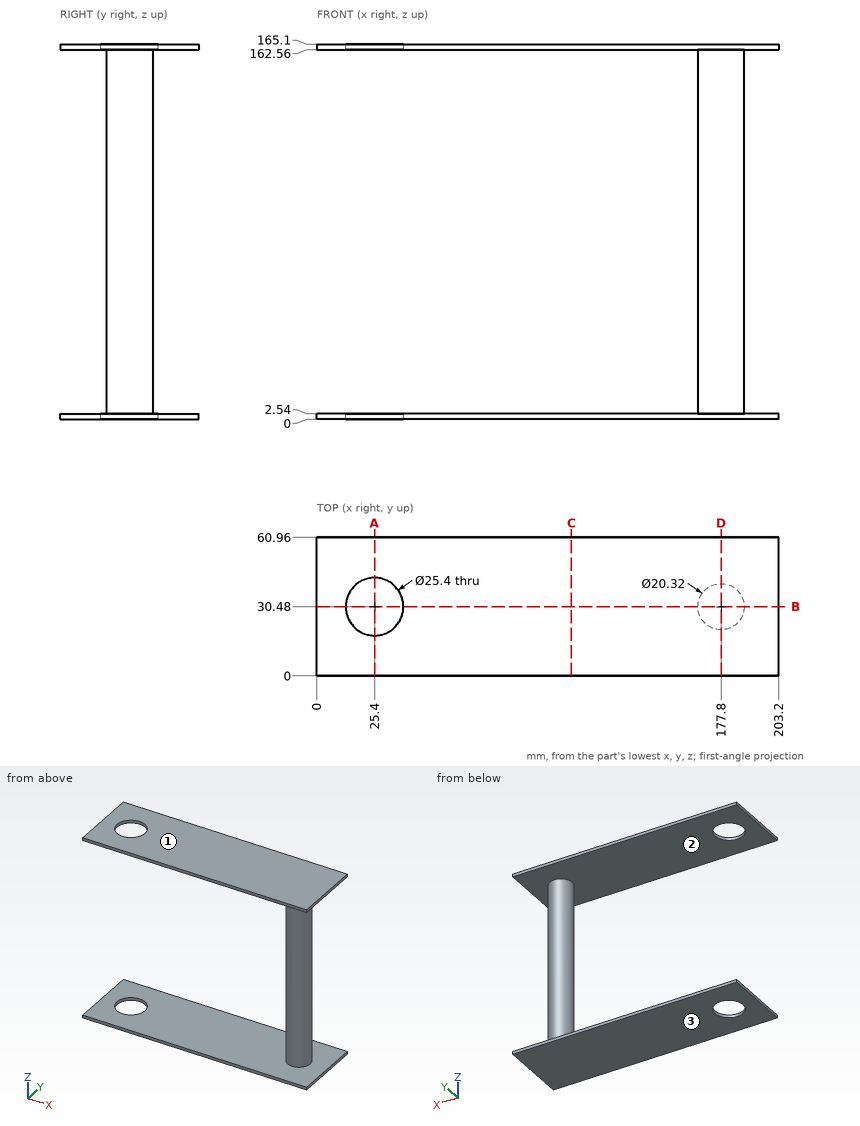
Study the drawing (mm; zero at the part's minimum x, y, z) and answer. Give positions to 0.01 mm unless a question says otherwise; leave off trailing zeros. Write each loop counter-clockwise with the first axis right and the second up, starting at its lowest first coordinate (ties: lowest second). Pieces come first, ordered by that corner, then holes. Notation, with made-up numbers: (49, 11.25) -> (74, 11.25) arc R13 cw to (74, 24.25) -> close; hole circle Ø6 at (-32.75, 51). An arc over 180 degrees is marked (long way). Answer in a Markdown table with one row per item.
1) Straight lines are drawn through the part: line 1 (Z direction, x = 170, y = 4); line 2 (Y direction, x = 25, z = 164); line 3 (X direction, y = 30, z = 1). For each, find the intervals that lie inside material, in ascending order. Write a range as [from, to].
Results list:
| item | result |
|---|---|
| line 1 | [0, 2.54], [162.56, 165.1] |
| line 2 | [0, 17.79], [43.17, 60.96] |
| line 3 | [0, 12.71], [38.09, 203.2] |
2) Section C-C on x = 112 is taken. Give the vertices of the cut face in (y, z).
Results list:
| item | result |
|---|---|
| outline | (0, 0) -> (60.96, 0) -> (60.96, 2.54) -> (0, 2.54) -> close; (0, 162.56) -> (60.96, 162.56) -> (60.96, 165.1) -> (0, 165.1) -> close |
3) Section B-B on y = 30.48 is taken. Give the vertices of the cut face in (x, z).
Results list:
| item | result |
|---|---|
| outline | (0, 0) -> (12.7, 0) -> (12.7, 2.54) -> (0, 2.54) -> close; (0, 162.56) -> (12.7, 162.56) -> (12.7, 165.1) -> (0, 165.1) -> close; (38.1, 0) -> (203.2, 0) -> (203.2, 2.54) -> (187.96, 2.54) -> (187.96, 162.56) -> (203.2, 162.56) -> (203.2, 165.1) -> (38.1, 165.1) -> (38.1, 162.56) -> (167.64, 162.56) -> (167.64, 2.54) -> (38.1, 2.54) -> close |
4) Each of these flat-tipped pins is pushed along its axis until it touches: pin 1 Ø20.5 at (x, y) = (25.4, 30.48) entering from +Z; pin 2 Ø5 at (y, z) = (25.5, 145) entering from +X. Where does it stop, or does it pass through?
Results list:
| item | result |
|---|---|
| pin 1 | through |
| pin 2 | x = 187.65 |
5) Section D-D on x = 177.8 is taken. Give the vertices of the cut face in (y, z).
Results list:
| item | result |
|---|---|
| outline | (0, 0) -> (60.96, 0) -> (60.96, 2.54) -> (40.64, 2.54) -> (40.64, 162.56) -> (60.96, 162.56) -> (60.96, 165.1) -> (0, 165.1) -> (0, 162.56) -> (20.32, 162.56) -> (20.32, 2.54) -> (0, 2.54) -> close |
6) Section A-A on x = 25.4 is taken. Give the vertices of the cut face in (y, z).
Results list:
| item | result |
|---|---|
| outline | (0, 0) -> (17.78, 0) -> (17.78, 2.54) -> (0, 2.54) -> close; (0, 162.56) -> (17.78, 162.56) -> (17.78, 165.1) -> (0, 165.1) -> close; (43.18, 0) -> (60.96, 0) -> (60.96, 2.54) -> (43.18, 2.54) -> close; (43.18, 162.56) -> (60.96, 162.56) -> (60.96, 165.1) -> (43.18, 165.1) -> close |
7) Determine the mould class of the marked faces 1, 2 and 3 for opening direction Z: released by +Z, released by -Z, zero draft, split by the parting line, or undercut.
Results list:
| item | result |
|---|---|
| face 1 | released by +Z |
| face 2 | undercut |
| face 3 | released by -Z |
